```python
from build123d import *
from OCP.BRepFilletAPI import BRepFilletAPI_MakeChamfer

# Parameters (mm, degrees)
SKETCH1_W           = 2.54
SKETCH1_H           = 2.54
BOSS_EXTRUDE1_DEPTH = 1.524
SKETCH2_W           = 0.508
SKETCH2_H           = 0.508
BOSS_EXTRUDE2_DEPTH = 6.35
SKETCH3_W           = 0.508
SKETCH3_H           = 0.508
BOSS_EXTRUDE3_DEPTH = 2.54
CHAMFER1_SIZE       = 0.508
CHAMFER1_SIZE2      = 0.1905
CHAMFER2_SIZE       = 0.508
CHAMFER2_SIZE2      = 0.1905
CHAMFER4_SIZE       = 0.3048
CHAMFER5_SIZE       = 0.3048


with BuildPart() as part:
    # Sketch1 → Boss-Extrude1 (new body)
    with BuildSketch(Plane(origin=(0, 0, 0), x_dir=(1, 0, 0), z_dir=(0, 1, 0))):
        with Locations((1.27, 1.27)):
            Rectangle(SKETCH1_W, SKETCH1_H)
    extrude(amount=BOSS_EXTRUDE1_DEPTH)

    # Sketch2 → Boss-Extrude2 (add)
    with BuildSketch(Plane(origin=(0, 1.524, 0), x_dir=(1, 0, 0), z_dir=(0, 1, 0))):
        with Locations((1.27, 1.27)):
            Rectangle(SKETCH2_W, SKETCH2_H)
    extrude(amount=BOSS_EXTRUDE2_DEPTH)

    # Sketch3 → Boss-Extrude3 (add)
    with BuildSketch(Plane.XZ):
        with Locations((1.27, -1.27)):
            Rectangle(SKETCH3_W, SKETCH3_H)
    extrude(amount=BOSS_EXTRUDE3_DEPTH)

    # Chamfer1: one chamfer whose edges measure the first distance from different faces: ONE call of the kernel's chamfer builder (chamfer() names one face for all edges)
    chamfer1_edges_1 = [part.edges().sort_by_distance(p)[0] for p in [
        (1.016, 7.874, -1.27),
    ]]
    chamfer1_side_1 = [part.faces().sort_by_distance(p)[0] for p in [
        (1.016, 4.699, -1.27),
    ]]
    chamfer1_edges_2 = [part.edges().sort_by_distance(p)[0] for p in [
        (1.27, 7.874, -1.016),
    ]]
    chamfer1_side_2 = [part.faces().sort_by_distance(p)[0] for p in [
        (1.27, 4.699, -1.016),
    ]]
    chamfer1_edges_3 = [part.edges().sort_by_distance(p)[0] for p in [
        (1.524, 7.874, -1.27),
    ]]
    chamfer1_side_3 = [part.faces().sort_by_distance(p)[0] for p in [
        (1.524, 4.699, -1.27),
    ]]
    chamfer1_edges_4 = [part.edges().sort_by_distance(p)[0] for p in [
        (1.27, 7.874, -1.524),
    ]]
    chamfer1_side_4 = [part.faces().sort_by_distance(p)[0] for p in [
        (1.27, 4.699, -1.524),
    ]]
    chamfer1 = BRepFilletAPI_MakeChamfer(part.part.solid().wrapped)
    for e in chamfer1_edges_1:
        chamfer1.Add(CHAMFER1_SIZE, CHAMFER1_SIZE2, e.wrapped, chamfer1_side_1[0].wrapped)  # the first distance lies on this face
    for e in chamfer1_edges_2:
        chamfer1.Add(CHAMFER1_SIZE, CHAMFER1_SIZE2, e.wrapped, chamfer1_side_2[0].wrapped)  # the first distance lies on this face
    for e in chamfer1_edges_3:
        chamfer1.Add(CHAMFER1_SIZE, CHAMFER1_SIZE2, e.wrapped, chamfer1_side_3[0].wrapped)  # the first distance lies on this face
    for e in chamfer1_edges_4:
        chamfer1.Add(CHAMFER1_SIZE, CHAMFER1_SIZE2, e.wrapped, chamfer1_side_4[0].wrapped)  # the first distance lies on this face
    add(Compound.cast(chamfer1.Shape()), mode=Mode.REPLACE)

    # Chamfer2: one chamfer whose edges measure the first distance from different faces: ONE call of the kernel's chamfer builder (chamfer() names one face for all edges)
    chamfer2_edges_1 = [part.edges().sort_by_distance(p)[0] for p in [
        (1.27, -2.54, -1.524),
    ]]
    chamfer2_side_1 = [part.faces().sort_by_distance(p)[0] for p in [
        (1.27, -1.27, -1.524),
    ]]
    chamfer2_edges_2 = [part.edges().sort_by_distance(p)[0] for p in [
        (1.524, -2.54, -1.27),
    ]]
    chamfer2_side_2 = [part.faces().sort_by_distance(p)[0] for p in [
        (1.524, -1.27, -1.27),
    ]]
    chamfer2_edges_3 = [part.edges().sort_by_distance(p)[0] for p in [
        (1.27, -2.54, -1.016),
    ]]
    chamfer2_side_3 = [part.faces().sort_by_distance(p)[0] for p in [
        (1.27, -1.27, -1.016),
    ]]
    chamfer2_edges_4 = [part.edges().sort_by_distance(p)[0] for p in [
        (1.016, -2.54, -1.27),
    ]]
    chamfer2_side_4 = [part.faces().sort_by_distance(p)[0] for p in [
        (1.016, -1.27, -1.27),
    ]]
    chamfer2 = BRepFilletAPI_MakeChamfer(part.part.solid().wrapped)
    for e in chamfer2_edges_1:
        chamfer2.Add(CHAMFER2_SIZE, CHAMFER2_SIZE2, e.wrapped, chamfer2_side_1[0].wrapped)  # the first distance lies on this face
    for e in chamfer2_edges_2:
        chamfer2.Add(CHAMFER2_SIZE, CHAMFER2_SIZE2, e.wrapped, chamfer2_side_2[0].wrapped)  # the first distance lies on this face
    for e in chamfer2_edges_3:
        chamfer2.Add(CHAMFER2_SIZE, CHAMFER2_SIZE2, e.wrapped, chamfer2_side_3[0].wrapped)  # the first distance lies on this face
    for e in chamfer2_edges_4:
        chamfer2.Add(CHAMFER2_SIZE, CHAMFER2_SIZE2, e.wrapped, chamfer2_side_4[0].wrapped)  # the first distance lies on this face
    add(Compound.cast(chamfer2.Shape()), mode=Mode.REPLACE)

    # Chamfer4
    chamfer4_edges = [part.edges().sort_by_distance(p)[0] for p in [
        (2.54, 1.524, -1.27),
        (1.27, 1.524, -2.54),
        (0, 1.524, -1.27),
        (1.27, 1.524, 0),
    ]]
    chamfer(chamfer4_edges, length=CHAMFER4_SIZE)

    # Chamfer5
    chamfer5_edges = [part.edges().sort_by_distance(p)[0] for p in [
        (1.27, 0, -2.54),
        (2.54, 0, -1.27),
        (1.27, 0, 0),
        (0, 0, -1.27),
    ]]
    chamfer(chamfer5_edges, length=CHAMFER5_SIZE)


solid = part.part
```
Input: part model. Units: mm. Frame: model coordinates. Give positions to 0.01 mm unless a question says otherwise; leave off trailing zeros. Loops run counter-clockwise (first coordinate to the right, second up) from the corner with the lowest first, then second, coordinate; pieces in that order, holes last.
1) Section query A-A on z = -0.55. Return the cut outline in (x, y), and give its area (3 significant figures).
A:
outline: (0, 0.3) - (0.3, 0) - (2.24, 0) - (2.54, 0.3) - (2.54, 1.22) - (2.24, 1.52) - (0.3, 1.52) - (0, 1.22) - close
area: 3.69 mm2
2) Section query B-B on x = 1.8. Return the cut outline in (y, z), and give its area (3 significant figures).
A:
outline: (0, -2.24) - (0.3, -2.54) - (1.22, -2.54) - (1.52, -2.24) - (1.52, -0.3) - (1.22, 0) - (0.3, 0) - (0, -0.3) - close
area: 3.69 mm2
3) Line query: L1, parallel to Y at x = 1.3, z = -2.15; L2, parallel to Z at x = 1.4, y = 7; L3, parallel to Y at x = 2.35, z = -1.3. Output: solid intervals per line, ascending.
A:
L1: y = 0 to 1.52
L2: z = -1.52 to -1.02
L3: y = 0.11 to 1.41
4) Section query C-C on y = 2. Return the cut outline in (x, z), and give its area (3 significant figures).
A:
outline: (1.02, -1.52) - (1.52, -1.52) - (1.52, -1.02) - (1.02, -1.02) - close
area: 0.258 mm2
5) Contact query for flat-ended pins moving along their axis: pin 1 (0.6 mm diameter, centred on x = 1.5, z = -1.5, fed in from +Y); pin 2 (0.6 mm diameter, centred on x = 1, y = 4, fed in from -Z); pin 3 (0.6 mm diameter, centred on y = 4, z = -1, fed in from +X). Output: stop coordinate, or through.
A:
pin 1: stops at y = 7.87
pin 2: stops at z = -1.52
pin 3: stops at x = 1.52
